Autodesk Inventor part; units mm, degrees
ref_plane "YZ Plane" through (0, 0, 0) normal (1, 0, 0) x (0, 1, 0)
ref_plane "XZ Plane" through (0, 0, 0) normal (0, 1, 0) x (-1, 0, 0)
ref_plane "XY Plane" through (0, 0, 0) normal (0, 0, 1) x (1, 0, 0)
sketch "Sketch1" plane through (0, 0, 0) normal (0, 0, 1) x (1, 0, 0)
  circle A0 centre (0, 0) radius 6.15
  line L0 (-31.1793, -0.1) -> (31.1793, -0.1)
  line L1 (31.1793, -0.1) -> (31.1793, 0.1)
  line L2 (31.1793, 0.1) -> (-31.1793, 0.1)
  line L3 (-31.1793, 0.1) -> (-31.1793, -0.1)
  line L4 (-31.1793, -0.1) -> (31.1793, 0.1) construction
  line L5 (31.1793, -0.1) -> (-31.1793, 0.1) construction
  line L6 (-18, 4) -> (18, 4)
  line L7 (18, 4) -> (18, 0)
  line L8 (18, 0) -> (-18, 0)
  line L9 (-18, 0) -> (-18, 4)
  circle A1 centre (0, 0) radius 10.15
  line L10 (0, 0) -> (0, 10.15) construction
  line L11 (-14, 0) -> (14, 0) construction
  point P0 (0, 6.15)
  point P1 (18, 0.1)
  point P2 (9.3286, 4)
  point P3 (-9.3286, 4)
  point P4 (-18, 0.1)
  point P5 (-6.1492, 0.1)
  point P6 (6.1492, 0.1)
  dimension "d0" = 12.3
  dimension "d1" = 0.2
  dimension "d2" = 4
  dimension "d3" = 4
  dimension "d6" = 28
  dimension "d7" = 4
extrude "Extrusion1" add sketch "Sketch1" along normal blind 6.5 contours A0 L6 A1 L2 | A0 L6 A1 | A1 L6 L7 L2 | L2 A1 L6 A0 | L2 L9 L6 A1
sketch "Sketch2" plane through (9.3286, 4, 0) normal (0, 1, 0) x (1, 0, 0)
  line L0 (-18.6572, 0) -> (-18.6572, -6.5) construction
  line L1 (0, 0) -> (0, -6.5) construction
  line L2 (0, -3.25) -> (4.6714, -3.25) construction
  line L3 (-18.6572, -3.25) -> (-23.3286, -3.25) construction
  point P0 (-9.3286, 0)
  dimension "d8" = 28
hole "Hole1" at (-14, 4, 3.25) at (14, 4, 3.25) direction (0, -1, 0) diameter 3.4 depth 8
fillet "Fillet1" radius 2 6 edges at (-18, 2.05, 0) (-18, 2.05, 6.5) (18, 2.05, 0) (18, 2.05, 6.5) (9.3286, 4, 3.25) (-9.3286, 4, 3.25)
chamfer "Chamfer1" distance 0.25 angle 45 33 edges at (0, 10.15, 6.5) (-9.559, 4.2715, 6.5) (-13.2826, 4, 6.5) (-17.4142, 4, 5.9142) (-18, 4, 3.25) (-17.4142, 4, 0.5858) (-13.2826, 4, 0) (-9.559, 4.2715, 0) (0, 10.15, 0) (9.559, 4.2715, 0) (13.2826, 4, 0) (17.4142, 4, 0.5858) (18, 4, 3.25) (17.4142, 4, 5.9142) (13.2826, 4, 6.5) (9.559, 4.2715, 6.5) (0, 6.15, 6.5) (-11.0746, 0.1, 6.5) (-17.4142, 0.1, 5.9142) (-18, 0.1, 3.25) (-17.4142, 0.1, 0.5858) (-11.0746, 0.1, 0) (11.0746, 0.1, 6.5) (17.4142, 0.1, 5.9142) (18, 0.1, 3.25) (17.4142, 0.1, 0.5858) (11.0746, 0.1, 0) (6.1492, 0.1, 3.25) (-6.1492, 0.1, 3.25) (14, 4, 1.55) (-14, 4, 1.55) (14, 0.1, 1.55) (-14, 0.1, 1.55)
properties part number "Idler-Clamp"
Build history of the part. All positions in model axes, mm. A direction names the side the tool comes from. Give positions to 0.01 mm unless a question says otherwise; leave off trailing zeros. Loops run counter-clockwise (first coordinate to the right, second up) from the corner with the lowest first, then second, coordinate; pieces in that order, holes last. Notation, with made-up numbers: (40, -27) -> (49, -27) arc R29 ccw to (49, 5) -> close; hole circle Ø11 at (15.25, 64). An arc over 180 degrees is marked (long way). Answer in a Markdown table with one row per item.
Item 1: Tool access for faces 1 (the cylindrical face through (-14.51, 2.03, 4.87)), 2 (the flat face through (-14, 4, 1)): list every direction of +Z, -Z, +X, -X, +Y, -Y with a clear straight run to the whole face (end or side of a thin tool).
Findings below:
| item | result |
|---|---|
| face 1 | +Y, -Y |
| face 2 | +Z, -Z, -X, +Y |
Item 2: Slice it at C-C on x = 0. Write the cut outline in (y, z).
Findings below:
| item | result |
|---|---|
| outline | (6.15, 0) -> (9.9, 0) -> (10.15, 0.25) -> (10.15, 6.25) -> (9.9, 6.5) -> (6.4, 6.5) -> (6.15, 6.25) -> close |
Item 3: Flat gauge pins, fed straight in: P1, Ø2, axis at x = -9.5, y = 6.5, coming from the +Z side; P2, Ø2, axis at x = 4, z = 3, coming from the -Y side; P3, Ø3, axis at x = -7, z = 4, coming from the +Y side; P4, Ø1.8, axis at x = -13, z = 2.5, coming from the +Y side. Where does each tip first touch, or does it go through?
Findings below:
| item | result |
|---|---|
| P1 | passes through |
| P2 | stops at y = 3.58 |
| P3 | stops at y = 8.53 |
| P4 | stops at y = 4 |
Item 4: Slice it at A-A on x = -14. Write the cut outline in (y, z).
Findings below:
| item | result |
|---|---|
| outline | (0.1, 0.25) -> (0.35, 0) -> (3.75, 0) -> (4, 0.25) -> (4, 1.3) -> (3.75, 1.55) -> (0.35, 1.55) -> (0.1, 1.3) -> close; (0.1, 5.2) -> (0.35, 4.95) -> (3.75, 4.95) -> (4, 5.2) -> (4, 6.25) -> (3.75, 6.5) -> (0.35, 6.5) -> (0.1, 6.25) -> close |
Item 5: Mould opens along X. For faces 3 (the cylindrical face through (-17.43, 2.07, 5.9)), 4 (the cylindrical face through (13.49, 2.03, 4.87)), 5 (the flat face through (11, 0.1, 3)) say: pulls with the +X half, pulls with the -X half, needs draft (parallel to the pull), parting line crosses it, or undercut.
Findings below:
| item | result |
|---|---|
| face 3 | pulls with the -X half |
| face 4 | undercut |
| face 5 | needs draft |
Item 6: Probe line 1 along X through (y, z) = (1.8, 3.25); line 2 along Z through (x, y) = (14, 1.05); line 3 along Y through (x, z) = (11, 5.5). List the from-to ranges inside material, lowest first. Write a range as [from, to].
Findings below:
| item | result |
|---|---|
| line 1 | x = [-18, -15.7], [-12.3, -5.88], [5.88, 12.3], [15.7, 18] |
| line 2 | z = [0, 1.55], [4.95, 6.5] |
| line 3 | y = [0.1, 4] |
Item 7: Slice it at B-B on z = 3.25. Give the number of separate pieces and of enclosed holes in the cut face, plus the area to 3 significant figures.
Findings below:
| item | result |
|---|---|
| separate pieces | 3 |
| enclosed holes | 0 |
| area | 139 mm² |
